from build123d import *

# Parameters (mm, degrees)
F1_DEPTH = 18
F2_R     = 300
F3_W     = 800
F3_H     = 850
F4_DEPTH = 18.001
F5_R     = 200


with BuildPart() as f1:
    # F0 (on Front) → F1 (new body)
    with BuildSketch(Plane.XZ):
        with BuildLine():
            Line((-685, 200), (-685, 0))
            Line((-685, 0), (685, 0))
            Line((685, 0), (685, 200))
            ThreePointArc((685, 200), (673.746048, 800.421727), (640, 1400))
            ThreePointArc((640, 1400), (0, 1500), (-640, 1400))
            ThreePointArc((-640, 1400), (-673.746048, 800.421727), (-685, 200))
        make_face()
    extrude(amount=F1_DEPTH)

    # F2
    f2_edges = [f1.edges().sort_by_distance(p)[0] for p in [
        (-640, -9, 1400),
        (640, -9, 1400),
    ]]
    fillet(f2_edges, radius=F2_R)

    # F3 (on face) → F4 (cut, through all)
    with BuildSketch(Plane.XZ.offset(18)):
        with Locations((0, 850)):
            Rectangle(F3_W, F3_H)
    extrude(amount=-F4_DEPTH, mode=Mode.SUBTRACT)

    # F5
    f5_edges = [f1.edges().sort_by_distance(p)[0] for p in [
        (-400, -9, 425),
        (-400, -9, 1275),
        (400, -9, 425),
        (400, -9, 1275),
    ]]
    fillet(f5_edges, radius=F5_R)


solid = f1.part
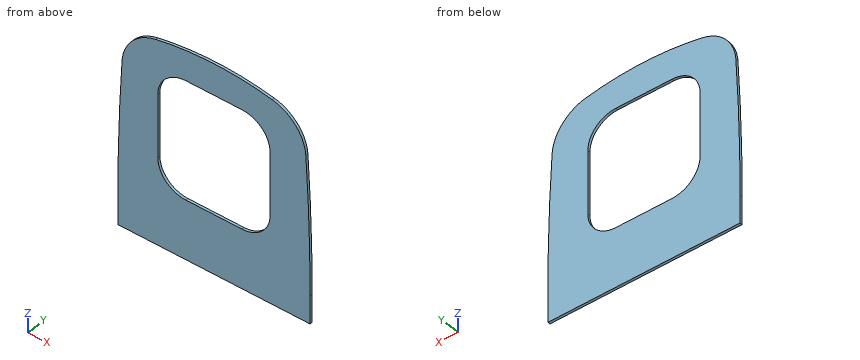
Check sheet for the modelled part. Datum: model origin and axes. Units: mm. Give positions to 0.01 mm unless a question says otherwise; leave off trailing zeros. Write each loop counter-clockwise with the first axis right and the second up, starting at its lowest first coordinate (ties: lowest second). Pieces come first, ordered by that corner, then holes. Notation, with made-up numbers: (3.5, 37.25) -> (14.5, 37.25) arc R19 ccw to (14.5, 62.25) -> close; hole circle Ø6 at (47.5, 35). An arc over 180 degrees is marked (long way). Write item = value, one per line.
Item 1: Sectioned sample at A-A on z = 915.5. Record the boundary of the cut face in (x, y), and give its area (3 significant figures).
Output:
outline = (-669.02, -18) -> (-400, -18) -> (-400, 0) -> (-669.02, 0) -> close; (400, -18) -> (669.02, -18) -> (669.02, 0) -> (400, 0) -> close
area = 9,680 mm^2
Item 2: Scan lines: probe 1 along Z at (x, y) = (150, -15.5); probe 2 along X at (y, z) = (-6.5, 481); probe 3 along Z at (x, y) = (363, -16.5). Record each from-to range of solid material in increasing order. Write a range as from..to.
Output:
probe_1 = 0..425, 1275..1494.63
probe_2 = -682.54..-338.79, 338.79..682.54
probe_3 = 0..509.11, 1190.89..1468.36
Item 3: Sectioned sample at B-B on x = -13. Record the boundary of the cut face in (y, z).
Output:
outline = (-18, 0) -> (0, 0) -> (0, 425) -> (-18, 425) -> close; (-18, 1275) -> (0, 1275) -> (0, 1499.96) -> (-18, 1499.96) -> close
Item 4: Gauge pin test, flat end, axial feed: pin 1 (10 mm diameter, centred on x = -460, y = -5.5, fed in from +Z). Record the tip position at first contact, or that the pin passes through.
Output:
pin_1 = 1447.51
